Read the model definition and answer for the solid it produces. Units are mm, in the model's axes. A direction names the side the tool comes from. Coordinates: 2 decimals unless noted, no trailing zeros. Order: outer loops, then holes, each group sorted by start corner. A loop starts at its lowest first (then second) coordinate and runs counter-clockwise, first axis right, second up.
from build123d import *

# Parameters (mm, degrees)
F1_DEPTH     = 2
F2_W         = 23.3004903048
F2_H         = 1.3265815725
F3_DEPTH     = 2
F2_W_2       = 24.5004919916
F2_H_2       = 2.5265832593
F4_DEPTH     = 3
F5_T1_DEPTH  = 29.5004919916
F5_T3_DEPTH  = 59.5122700134
F5_T5_DEPTH  = 5.0265832593
F5_T7_DEPTH  = 30.4185097339
F5_T9_DEPTH  = 18.246874844
F5_T11_DEPTH = 29.5004919916
F5_T17_DEPTH = 7.5265832593
F5_T21_DEPTH = 32.9185097339
F5_T28_DEPTH = 32.9185097339
F5_T32_DEPTH = 7.5265832593
F5_T39_DEPTH = 20.746874844
F5_T43_DEPTH = 32.9185097339
F5_T50_DEPTH = 32.9185097339
F5_T54_DEPTH = 20.746874844


# Not quite as in the source:
# - a fillet or chamfer that OpenCascade refuses, or shapes differently, is made with other operations: its cross-section is extruded or revolved along the edge and cut away or added


with BuildPart() as f1:
    # F0 (on Top) → F1 (new body)
    with BuildSketch(Plane.XY):
        Polygon((25.1509650471, -26.6069659193), (25.1509650471, 27.9053040941), (0.6504730554, 27.9053040941), (0.6504730554, 25.3787208349), (-29.7680366784, 25.3787208349), (-29.7680366784, 27.9053040941), (-54.2685286701, 27.9053040941), (-54.2685286701, -26.6069659193), (-29.7680366784, -26.6069659193), (-29.7680366784, -10.8600910753), (0.6504730554, -10.8600910753), (0.6504730554, -26.6069659193), align=None)
    extrude(amount=F1_DEPTH)

    # F0 (on Top) + F2 (on face) → F3 (cut)
    with BuildSketch(Plane.XY):
        Polygon((25.1509650471, -26.6069659193), (25.1509650471, 27.9053040941), (0.6504730554, 27.9053040941), (0.6504730554, 25.3787208349), (-29.7680366784, 25.3787208349), (-29.7680366784, 27.9053040941), (-54.2685286701, 27.9053040941), (-54.2685286701, -26.6069659193), (-29.7680366784, -26.6069659193), (-29.7680366784, -10.8600910753), (0.6504730554, -10.8600910753), (0.6504730554, -26.6069659193), align=None)
    with BuildSketch(Plane.XY.offset(2)):
        with Locations((-42.0182826743, 26.6420124645)):
            Rectangle(F2_W, F2_H)
    extrude(amount=-F3_DEPTH, mode=Mode.SUBTRACT)

    # F2 (on face) → F4 (join)
    with BuildSketch(Plane.XY.offset(2)):
        with Locations((-42.0182826743, 26.6420124645)):
            Rectangle(F2_W_2, F2_H_2)
        with Locations((-42.0182826743, 26.6420124645)):
            Rectangle(F2_W, F2_H, mode=Mode.SUBTRACT)
    extrude(amount=F4_DEPTH)

    # F5: fillet of radius 1 on 12 edges, made by hand

    # F5_s2 → F5_t1 (cut)
    with BuildSketch(Plane.YZ.offset(-56.7685286701)):
        with BuildLine():
            ThreePointArc((-25.6069659193, 0), (-26.3140727005, 0.2928932188), (-26.6069659193, 1))
            Line((-26.6069659193, 1), (-26.6069659193, 0))
            Line((-26.6069659193, 0), (-25.6069659193, 0))
        make_face()
        with BuildLine():
            ThreePointArc((26.9053040941, 0), (27.6124108753, 0.2928932188), (27.9053040941, 1))
            Line((27.9053040941, 1), (27.9053040941, 0))
            Line((27.9053040941, 0), (26.9053040941, 0))
        make_face()
    extrude(amount=F5_T1_DEPTH, mode=Mode.SUBTRACT)

    # F5_s4 → F5_t3 (cut)
    with BuildSketch(Plane.XZ.offset(-30.4053040941)):
        with BuildLine():
            ThreePointArc((-54.2685286701, 1), (-53.9756354513, 0.2928932188), (-53.2685286701, 0))
            Line((-53.2685286701, 0), (-54.2685286701, 0))
            Line((-54.2685286701, 0), (-54.2685286701, 1))
        make_face()
        with BuildLine():
            ThreePointArc((24.1509650471, 0), (24.8580718283, 0.2928932188), (25.1509650471, 1))
            Line((25.1509650471, 1), (25.1509650471, 0))
            Line((25.1509650471, 0), (24.1509650471, 0))
        make_face()
    extrude(amount=F5_T3_DEPTH, mode=Mode.SUBTRACT)

    # F5_s6 → F5_t5 (cut)
    with BuildSketch(Plane.XZ.offset(-30.4053040941)):
        with BuildLine():
            ThreePointArc((-30.7680366784, 0), (-30.0609298972, 0.2928932188), (-29.7680366784, 1))
            Line((-29.7680366784, 1), (-29.7680366784, 0))
            Line((-29.7680366784, 0), (-30.7680366784, 0))
        make_face()
        with BuildLine():
            ThreePointArc((1.6504730554, 0), (0.9433662742, 0.2928932188), (0.6504730554, 1))
            Line((0.6504730554, 1), (0.6504730554, 0))
            Line((0.6504730554, 0), (1.6504730554, 0))
        make_face()
    extrude(amount=F5_T5_DEPTH, mode=Mode.SUBTRACT)

    # F5_s8 → F5_t7 (cut)
    with BuildSketch(Plane.YZ.offset(-29.7680366784)):
        with BuildLine():
            ThreePointArc((24.3787208349, 0), (25.085827616, 0.2928932188), (25.3787208349, 1))
            Line((25.3787208349, 1), (25.3787208349, 0))
            Line((25.3787208349, 0), (24.3787208349, 0))
        make_face()
        with BuildLine():
            ThreePointArc((-9.8600910753, 0), (-10.5671978565, 0.2928932188), (-10.8600910753, 1))
            Line((-10.8600910753, 1), (-10.8600910753, 0))
            Line((-10.8600910753, 0), (-9.8600910753, 0))
        make_face()
    extrude(amount=F5_T7_DEPTH, mode=Mode.SUBTRACT)

    # F5_s10 → F5_t9 (cut)
    with BuildSketch(Plane.XZ.offset(10.8600910753)):
        with BuildLine():
            ThreePointArc((-30.7680366784, 0), (-30.0609298972, 0.2928932188), (-29.7680366784, 1))
            Line((-29.7680366784, 1), (-29.7680366784, 0))
            Line((-29.7680366784, 0), (-30.7680366784, 0))
        make_face()
        with BuildLine():
            ThreePointArc((1.6504730554, 0), (0.9433662742, 0.2928932188), (0.6504730554, 1))
            Line((0.6504730554, 1), (0.6504730554, 0))
            Line((0.6504730554, 0), (1.6504730554, 0))
        make_face()
    extrude(amount=F5_T9_DEPTH, mode=Mode.SUBTRACT)

    # F5_s12 → F5_t11 (cut)
    with BuildSketch(Plane.YZ.offset(-1.8495269446)):
        with BuildLine():
            ThreePointArc((-25.6069659193, 0), (-26.3140727005, 0.2928932188), (-26.6069659193, 1))
            Line((-26.6069659193, 1), (-26.6069659193, 0))
            Line((-26.6069659193, 0), (-25.6069659193, 0))
        make_face()
        with BuildLine():
            ThreePointArc((26.9053040941, 0), (27.6124108753, 0.2928932188), (27.9053040941, 1))
            Line((27.9053040941, 1), (27.9053040941, 0))
            Line((27.9053040941, 0), (26.9053040941, 0))
        make_face()
    extrude(amount=F5_T11_DEPTH, mode=Mode.SUBTRACT)


with BuildPart() as f5_tool15:
    # F5_s16 → F5_t17 (new body)
    with BuildSketch(Plane.XZ.offset(-22.8787208349)):
        with BuildLine():
            ThreePointArc((-30.7680366784, 0), (-30.0609298972, 0.2928932188), (-29.7680366784, 1))
            Line((-29.7680366784, 1), (-29.7680366784, 0))
            Line((-29.7680366784, 0), (-30.7680366784, 0))
        make_face()
    extrude(amount=-F5_T17_DEPTH)

    split(bisect_by=Plane.XZ.offset(-25.3787208349), keep=Keep.TOP)


with BuildPart() as f5_tool19:
    # F5_s20 → F5_t21 (new body)
    with BuildSketch(Plane.YZ.offset(0.6504730554)):
        with BuildLine():
            ThreePointArc((24.3787208349, 0), (25.085827616, 0.2928932188), (25.3787208349, 1))
            Line((25.3787208349, 1), (25.3787208349, 0))
            Line((25.3787208349, 0), (24.3787208349, 0))
        make_face()
    extrude(amount=-F5_T21_DEPTH)

    split(bisect_by=Plane.YZ.offset(-29.7680366784), keep=Keep.BOTTOM)


with BuildPart() as f5_tool15_1:
    add(f5_tool15.part)

    # F5_t23: intersect F5_tool19
    add(f5_tool19.part, mode=Mode.INTERSECT)


with BuildPart() as f1_1:
    add(f1.part)

    # F5_t13: cut F5_tool15
    add(f5_tool15_1.part, mode=Mode.SUBTRACT)


with BuildPart() as f5_tool26:
    # F5_s27 → F5_t28 (new body)
    with BuildSketch(Plane.YZ.offset(3.1504730554)):
        with BuildLine():
            ThreePointArc((24.3787208349, 0), (25.085827616, 0.2928932188), (25.3787208349, 1))
            Line((25.3787208349, 1), (25.3787208349, 0))
            Line((25.3787208349, 0), (24.3787208349, 0))
        make_face()
    extrude(amount=-F5_T28_DEPTH)

    split(bisect_by=Plane.YZ.offset(0.6504730554), keep=Keep.TOP)


with BuildPart() as f5_tool30:
    # F5_s31 → F5_t32 (new body)
    with BuildSketch(Plane.XZ.offset(-30.4053040941)):
        with BuildLine():
            ThreePointArc((1.6504730554, 0), (0.9433662742, 0.2928932188), (0.6504730554, 1))
            Line((0.6504730554, 1), (0.6504730554, 0))
            Line((0.6504730554, 0), (1.6504730554, 0))
        make_face()
    extrude(amount=F5_T32_DEPTH)

    split(bisect_by=Plane.XZ.offset(-25.3787208349), keep=Keep.TOP)


with BuildPart() as f5_tool26_1:
    add(f5_tool26.part)

    # F5_t34: intersect F5_tool30
    add(f5_tool30.part, mode=Mode.INTERSECT)


with BuildPart() as f1_2:
    add(f1_1.part)

    # F5_t24: cut F5_tool26
    add(f5_tool26_1.part, mode=Mode.SUBTRACT)


with BuildPart() as f5_tool37:
    # F5_s38 → F5_t39 (new body)
    with BuildSketch(Plane.XZ.offset(29.1069659193)):
        with BuildLine():
            ThreePointArc((-30.7680366784, 0), (-30.0609298972, 0.2928932188), (-29.7680366784, 1))
            Line((-29.7680366784, 1), (-29.7680366784, 0))
            Line((-29.7680366784, 0), (-30.7680366784, 0))
        make_face()
    extrude(amount=-F5_T39_DEPTH)

    split(bisect_by=Plane.XZ.offset(10.8600910753), keep=Keep.BOTTOM)


with BuildPart() as f5_tool41:
    # F5_s42 → F5_t43 (new body)
    with BuildSketch(Plane.YZ.offset(-32.2680366784)):
        with BuildLine():
            ThreePointArc((-9.8600910753, 0), (-10.5671978565, 0.2928932188), (-10.8600910753, 1))
            Line((-10.8600910753, 1), (-10.8600910753, 0))
            Line((-10.8600910753, 0), (-9.8600910753, 0))
        make_face()
    extrude(amount=F5_T43_DEPTH)

    split(bisect_by=Plane.YZ.offset(-29.7680366784), keep=Keep.BOTTOM)


with BuildPart() as f5_tool37_1:
    add(f5_tool37.part)

    # F5_t45: intersect F5_tool41
    add(f5_tool41.part, mode=Mode.INTERSECT)


with BuildPart() as f1_3:
    add(f1_2.part)

    # F5_t35: cut F5_tool37
    add(f5_tool37_1.part, mode=Mode.SUBTRACT)


with BuildPart() as f5_tool48:
    # F5_s49 → F5_t50 (new body)
    with BuildSketch(Plane.YZ.offset(-29.7680366784)):
        with BuildLine():
            ThreePointArc((-9.8600910753, 0), (-10.5671978565, 0.2928932188), (-10.8600910753, 1))
            Line((-10.8600910753, 1), (-10.8600910753, 0))
            Line((-10.8600910753, 0), (-9.8600910753, 0))
        make_face()
    extrude(amount=F5_T50_DEPTH)

    split(bisect_by=Plane.YZ.offset(0.6504730554), keep=Keep.TOP)


with BuildPart() as f5_tool52:
    # F5_s53 → F5_t54 (new body)
    with BuildSketch(Plane.XZ.offset(8.3600910753)):
        with BuildLine():
            ThreePointArc((1.6504730554, 0), (0.9433662742, 0.2928932188), (0.6504730554, 1))
            Line((0.6504730554, 1), (0.6504730554, 0))
            Line((0.6504730554, 0), (1.6504730554, 0))
        make_face()
    extrude(amount=F5_T54_DEPTH)

    split(bisect_by=Plane.XZ.offset(10.8600910753), keep=Keep.BOTTOM)


with BuildPart() as f5_tool48_1:
    add(f5_tool48.part)

    # F5_t56: intersect F5_tool52
    add(f5_tool52.part, mode=Mode.INTERSECT)


with BuildPart() as f1_4:
    add(f1_3.part)

    # F5_t46: cut F5_tool48
    add(f5_tool48_1.part, mode=Mode.SUBTRACT)


solid = f1_4.part
Q1. Each of these flat-tipped pins is pushed along its axis until it touches: P1, Ø8, axis at x = -15.5, y = 19.5, coming from the +Z side; P2, Ø1.5, axis at x = -47, z = 3.5, coming from the -Y side; P3, Ø1.5, axis at y = 26.5, z = 3, coming from the +X side. Where does it stop, or does it pass through?
Q2. Straight lines are drawn through the part: L1, parallel to Y at x = -34.5, z = 3.2; L2, parallel to Y at x = -32.5, z = 1.95; L3, parallel to Z at x = -1, y = -3. For each, find the intervals that lie inside material, in ascending order.
Q3. The part is cut by section B-B, the plane x = -21.5. Determine the outline of the cut face in (y, z).
Q4. The part is cut by section A-A, the plane z = 4. Determine the outline of the cut face in (x, y), then the cut area to 3 significant figures.
Q5. Which of the six approach directions +Z, -Z, +X, -X, +Y, -Y give full straight-line access (tool end or side, diameter ignored) to faces 1 (the flat face through (-29.768, 27, 3)), 2 (the flat face through (-54.269, 2.5, 1.7)), 3 (the flat face through (-42, 25.379, 3))?
Q6. Determine the mould class of faces 4 (the flat face through (-42, 27.305, 3)), 5 (the flat face through (-15, 1, 0)), 6 (the flat face through (-42, 25.979, 2)), 7 (the flat face through (-42, 27.905, 3)) for opening direction Y: +Y half, -Y half, draft (parallel to the pull), parting line (faces both ways), or undercut.
Q7. The part is cut by section C-C, the plane y = 9. Determine the outline of the cut face in (x, z).
Computed values:
1. P1: stops at z = 2
1. P2: stops at y = 25.38
1. P3: stops at x = -29.77
2. L1: y = 25.38 to 25.98, 27.31 to 27.91
2. L2: y = -26.61 to 25.98, 27.31 to 27.91
2. L3: z = 0 to 2
3. outline: (-10.86, 1) arc R1 ccw to (-9.86, 0) - (24.38, 0) arc R1 ccw to (25.38, 1) - (25.38, 2) - (-10.86, 2) - close
4. outline: (-54.27, 25.38) - (-29.77, 25.38) - (-29.77, 27.91) - (-54.27, 27.91) - close; hole (-53.67, 25.98) - (-30.37, 25.98) - (-30.37, 27.31) - (-53.67, 27.31) - close
4. area: 31.0 mm2
5. face 1: +Z, -Z, +Y
5. face 2: +Z, -Z, -X, +Y, -Y
5. face 3: +Z, +X, -X, -Y
6. face 4: undercut
6. face 5: draft
6. face 6: undercut
6. face 7: +Y half
7. outline: (-54.27, 1) arc R1 ccw to (-53.27, 0) - (24.15, 0) arc R1 ccw to (25.15, 1) - (25.15, 2) - (-54.27, 2) - close
